Can you work these out from the model? Positions are in its coordinate system, mm. A direction names the side the tool comes from. Coordinates: 2 decimals unless noted, no trailing zeros. Order: outer loops, then holes, each group sorted by start corner. A loop starts at its lowest first (then second) coordinate and runs counter-clockwise, first axis right, second up. Notation, with made-up numbers: (25, -9.75) -> (77, -9.75) arc R23 cw to (77, 17.25) -> close; hole circle Ø9 at (-4, 34.25). An arc over 180 degrees is marked (long way). Answer in a Markdown table with one row per item. Add a question column.
1. We'd pull the mould along Y, two halves only. Please class faces 1 (the face through (3.92, 3.86, 2.03)), 2 (the face through (3.86, -3.92, 2.03)), 3 (the face through (1, -3, 2)): pulls with the +Y half, pulls with the -Y half, needs draft (parallel to the pull), parting line crosses it, or undercut.
2. On a 3-axis mill with a long thin cutter (end or side, diameter ignored), from which of +Z, -Z, +X, -X, +Y, -Y can I reach the whole of each face in a straight line? I mean faces 4 (the face through (3.233, -1.341, 2.986)), 5 (the face through (-3.92, -3.86, 2.03)). Say none if no direction works.
3. If I drill on line 1 along Y through (x, z) = (0, 3.5); line 2 along Y through (x, z) = (0, 0.7); line 3 along X through (y, z) = (0.5, 1.85), over which ranges is the centre line in solid material (lowest first)? Write a range as [from, to].
4. Imagine slicing it at B-B on y = 0. Write out the boundary of the cut face in (x, z).
5. Will this pin go through, and if not, where does the flat tip stop? pin 1 (6 mm diameter, centred on x = 0, y = 0, fed in from +Z).
6. Imagine slicing it at D-D on z = 2.4. Write out the boundary of the cut face in (x, y), plus the area to 3 significant figures.
7. Imagine slicing it at A-A on z = 1.25. Write out the boundary of the cut face in (x, y).
from build123d import *

# Parameters (mm, degrees)
F2_W     = 11.5
F2_H     = 11.5
F2_W_2   = 10.5
F2_H_2   = 10.5
F3_DEPTH = 25


with BuildPart() as f1:
    # F0 (on Front) → F1 (revolve)
    with BuildSketch(Plane.XZ):
        Polygon((5.5, 4), (3.5, 4), (3.5, 2), (2.7, 2), (2.7, 0), (5.5, 0), align=None)
    revolve(axis=Axis((0, 0, 5.877999), (0, 0, 1)))

    # F2 (on Top) → F3 (cut)
    with BuildSketch(Plane.XY):
        Rectangle(F2_W, F2_H)
        Rectangle(F2_W_2, F2_H_2, mode=Mode.SUBTRACT)
    extrude(amount=F3_DEPTH, mode=Mode.SUBTRACT)


solid = f1.part
Answers follow:
| question | item | result |
|---|---|---|
| 1 | face 1 | pulls with the +Y half |
| 1 | face 2 | pulls with the -Y half |
| 1 | face 3 | undercut |
| 2 | face 4 | +Z |
| 2 | face 5 | +Z, -Z, -X, -Y |
| 3 | line 1 | y = [-5.25, -3.5], [3.5, 5.25] |
| 3 | line 2 | y = [-5.25, -2.7], [2.7, 5.25] |
| 3 | line 3 | x = [-5.25, -2.65], [2.65, 5.25] |
| 4 | outline | (-5.25, 0) -> (-2.7, 0) -> (-2.7, 2) -> (-3.5, 2) -> (-3.5, 4) -> (-5.25, 4) -> close; (2.7, 0) -> (5.25, 0) -> (5.25, 4) -> (3.5, 4) -> (3.5, 2) -> (2.7, 2) -> close |
| 5 | pin 1 | stops at z = 2 |
| 6 | outline | (-5.25, -1.64) arc R5.5 ccw to (-1.64, -5.25) -> (1.64, -5.25) arc R5.5 ccw to (5.25, -1.64) -> (5.25, 1.64) arc R5.5 ccw to (1.64, 5.25) -> (-1.64, 5.25) arc R5.5 ccw to (-5.25, 1.64) -> close; hole circle Ø7 at (0, 0) |
| 6 | area | 54.4 mm² |
| 7 | outline | (-5.25, -1.64) arc R5.5 ccw to (-1.64, -5.25) -> (1.64, -5.25) arc R5.5 ccw to (5.25, -1.64) -> (5.25, 1.64) arc R5.5 ccw to (1.64, 5.25) -> (-1.64, 5.25) arc R5.5 ccw to (-5.25, 1.64) -> close; hole circle Ø5.4 at (0, 0) |
